Source: CAD feature listing. Evaluate the final solid. Frame: model axes, mm. Face numbers are marked on the shaded views. A direction names the side the tool comes from. Round coordinates to 2 decimals unless told otherwise and drop trailing zeros. Order: outer loops, then holes, each group sorted by start corner. A loop starts at its lowest first (then second) coordinate and runs counter-clockwise, first axis right, second up. Notation, with made-up numbers: (82, 80.25) -> (91, 80.25) arc R30 cw to (91, 108.25) -> close; hole circle Ø7 at (-28, 30). An arc over 180 degrees is marked (long way). Write item = value, one per line. Start each with the question number.
(1) Cut plane A-A on z = 22.5. Return the cut outline in (x, y) (3 decimals), then the cut area to 3 significant figures.
(2) Draft query along Y for the marked faces 4, 5 and 6. Return one class per face: released by +Y, released by -Y, zero draft, split by the parting line, or undercut.
(3) Cut plane C-C on y = 0. Return the cut outline in (x, z), then the cut area to 3 significant figures.
(4) Contact query for flat-ended pins moving along their axis: pin 1 Ø16 at (x, y) = (-2, -4.5) entering from +Z; pin 2 Ø12.5 at (x, z) = (-1, 15.5) entering from -Y; pin 3 Ø12 at (y, z) = (-6.5, 4.5) entering from +X; pin 4 Ø4 at (x, y) = (0, 16.5) entering from +Z. Output: stop coordinate, or through.
(5) Cut plane D-D on x = 0. Return the cut outline in (y, z) (3 decimals).
(6) Cut plane B-B on z = 11.75. Return the cut outline in (x, y), then the cut area to 3 significant figures.
(7) Reachability of the marked faces 1, 2 and 3 from +Z, -Z, +X, -X, +Y, -Y: full face, straight path, thin tool, end or side. Return the list, or none.
(8) Ray query, line 1 (Y direction, x = 0, z = 2.55) (3 decimals); line 2 (Z direction, x = 0, y = 23.6) (3 decimals); line 3 (Z direction, x = 0, y = -18). Return the intervals inside material, ascending.
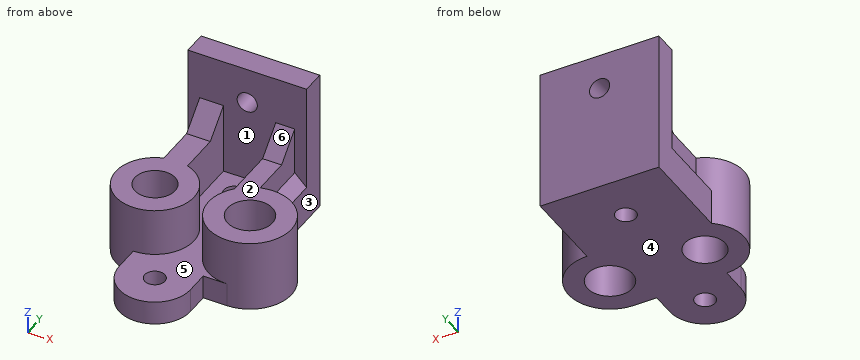
from build123d import *

# Parameters (mm, degrees)
F0_R          = 2.125
F0_R_2        = 4.25
F0_R_3        = 4.75
F1_DEPTH      = 5
F2_W          = 25
F2_H          = 5
F3_DEPTH      = 25
F4_R          = 8.25
F4_R_2        = 4.25
F4_R_3        = 8.75
F4_R_4        = 4.75
F5_DEPTH      = 10
F6_R          = 2.125
F7_DEPTH      = 5.001
F8_W          = 5
F8_H          = 13.6379074032
F8_W_2        = 4
F8_H_2        = 15.6423127431
F9_DEPTH      = 10
F10_T1_DEPTH  = 5
F10_T3_DEPTH  = 4
F10_T8_DEPTH  = 17.8584149398
F10_T13_DEPTH = 16.8584149398
F10_T18_DEPTH = 26.4963223431
F10_S19_R     = 8.25
F10_T20_DEPTH = 15
F10_T25_DEPTH = 26.4963223431
F10_S26_R     = 8.25
F10_T27_DEPTH = 15
F10_T32_DEPTH = 25.9731600242
F10_S34_R     = 8.75
F10_T35_DEPTH = 15


# Not quite as in the source:
# - a fillet or chamfer that OpenCascade refuses, or shapes differently, is made with other operations: its cross-section is extruded or revolved along the edge and cut away or added


with BuildPart() as f1:
    # F0 (on Top) → F1 (new body)
    with BuildSketch(Plane.XY):
        with BuildLine():
            Line((12.5, 26.5), (0, 26.5))
            Line((0, 26.5), (-12.5, 26.5))
            Line((-12.5, 26.5), (-12.5, 6.5622023742))
            ThreePointArc((-12.5, 6.5622023742), (-15.3166703137, -2.6385915194), (-7.5, -8.25))
            Line((-7.5, -8.25), (-7.5, -13.6))
            ThreePointArc((-7.5, -13.6), (-5.3033008589, -18.9033008589), (0, -21.1))
            ThreePointArc((0, -21.1), (5.3033008589, -18.9033008589), (7.5, -13.6))
            Line((7.5, -13.6), (7.5, -8.75))
            Line((7.5, -8.75), (12.5, -8.75))
            ThreePointArc((12.5, -8.75), (21.25, 0), (12.5, 8.75))
            Line((12.5, 8.75), (12.5, 26.5))
        make_face()
        with Locations((0, -13.6)):
            Circle(F0_R, mode=Mode.SUBTRACT)
        with Locations((-7.5, 0)):
            Circle(F0_R_2, mode=Mode.SUBTRACT)
        with Locations((12.5, 0)):
            Circle(F0_R_3, mode=Mode.SUBTRACT)
        with Locations((0, 16.5)):
            Circle(F0_R, mode=Mode.SUBTRACT)
    extrude(amount=F1_DEPTH)

    # F2 (on face) → F3 (join)
    with BuildSketch(Plane.XY.offset(5)):
        with Locations((0, 24)):
            Rectangle(F2_W, F2_H)
    extrude(amount=F3_DEPTH)

    # F4 (on face) → F5 (join)
    with BuildSketch(Plane.XY.offset(5)):
        with Locations((-7.5, 0)):
            Circle(F4_R)
        with Locations((-7.5, 0)):
            Circle(F4_R_2, mode=Mode.SUBTRACT)
        with Locations((12.5, 0)):
            Circle(F4_R_3)
        with Locations((12.5, 0)):
            Circle(F4_R_4, mode=Mode.SUBTRACT)
    extrude(amount=F5_DEPTH)

    # F6 (on face) → F7 (cut, through all)
    with BuildSketch(Plane.XZ.offset(-21.5)):
        with Locations((0, 22.5)):
            Circle(F6_R)
    extrude(amount=-F7_DEPTH, mode=Mode.SUBTRACT)

    # F8 (on face) → F9 (join)
    with BuildSketch(Plane.XY.offset(5)):
        with Locations((-7.5, 14.6810462984)):
            Rectangle(F8_W, F8_H)
        with Locations((8, 13.6788436285)):
            Rectangle(F8_W_2, F8_H_2)
    extrude(amount=F9_DEPTH)

    # F10: chamfer of 5 on 4 edges, made by hand

    # F10_s2 → F10_t1 (join)
    with BuildSketch(Plane.YZ.offset(-10)):
        Polygon((21.5, 20), (16.5, 15), (21.5, 15), align=None)
    extrude(amount=F10_T1_DEPTH)

    # F10_s4 → F10_t3 (join)
    with BuildSketch(Plane.YZ.offset(6)):
        Polygon((21.5, 20), (16.5, 15), (21.5, 15), align=None)
    extrude(amount=F10_T3_DEPTH)


with BuildPart() as f10_tool6:
    # F10_s7 → F10_t8 (new body)
    with BuildSketch(Plane.YZ.offset(7.8584149398)):
        Polygon((21.5, 20), (16.5, 15), (21.5, 15), align=None)
    extrude(amount=-F10_T8_DEPTH)

    split(bisect_by=Plane.YZ.offset(6), keep=Keep.TOP)


with BuildPart() as f1_1:
    add(f1.part)

    # F10_t5: union F10_tool6
    add(f10_tool6.part)


with BuildPart() as f10_tool11:
    # F10_s12 → F10_t13 (new body)
    with BuildSketch(Plane.YZ.offset(10)):
        Polygon((21.5, 20), (16.5, 15), (21.5, 15), align=None)
    extrude(amount=-F10_T13_DEPTH)

    split(bisect_by=Plane.YZ.offset(-5), keep=Keep.BOTTOM)


with BuildPart() as f1_2:
    add(f1_1.part)

    # F10_t10: union F10_tool11
    add(f10_tool11.part)


with BuildPart() as f10_tool16:
    # F10_s17 → F10_t18 (new body)
    with BuildSketch(Plane.XZ.offset(-21.5)):
        Polygon((-10, 10), (-15, 5), (-10, 5), align=None)
    extrude(amount=F10_T18_DEPTH)

    # F10_s19 → F10_t20 (cut, symmetric)
    with BuildSketch(Plane.XY.offset(7.5)):
        with Locations((-7.5, 0)):
            Circle(F10_S19_R)
    extrude(amount=F10_T20_DEPTH, both=True, mode=Mode.SUBTRACT)

    split(bisect_by=Plane.YZ.offset(-12.5), keep=Keep.TOP)


with BuildPart() as f1_3:
    add(f1_2.part)

    # F10_t15: union F10_tool16
    add(f10_tool16.part)


with BuildPart() as f10_tool23:
    # F10_s24 → F10_t25 (new body)
    with BuildSketch(Plane.XZ.offset(-21.5)):
        Polygon((-10, 10), (-15, 5), (-10, 5), align=None)
    extrude(amount=F10_T25_DEPTH)

    # F10_s26 → F10_t27 (intersect, symmetric)
    with BuildSketch(Plane.XY.offset(7.5)):
        with Locations((-7.5, 0)):
            Circle(F10_S26_R)
    extrude(amount=F10_T27_DEPTH, both=True, mode=Mode.INTERSECT)

    split(bisect_by=Plane.YZ.offset(-12.5), keep=Keep.BOTTOM)


with BuildPart() as f1_4:
    add(f1_3.part)

    # F10_t22: union F10_tool23
    add(f10_tool23.part)


with BuildPart() as f10_tool30:
    # F10_s31 → F10_t32 (new body)
    with BuildSketch(Plane.XZ.offset(4.4731600242)):
        Polygon((15, 5), (10, 10), (10, 5), align=None)
    extrude(amount=-F10_T32_DEPTH)

    split(bisect_by=Plane.YZ.offset(12.5), keep=Keep.BOTTOM)

    # F10_s34 → F10_t35 (cut, symmetric)
    with BuildSketch(Plane.XY.offset(7.5)):
        with Locations((12.5, 0)):
            Circle(F10_S34_R)
    extrude(amount=F10_T35_DEPTH, both=True, mode=Mode.SUBTRACT)


with BuildPart() as f1_5:
    add(f1_4.part)

    # F10_t29: union F10_tool30
    add(f10_tool30.part)


solid = f1_5.part
Evaluation:
q1.outline = (-12.5, 21.5) -> (-2.125, 21.5) -> (-2.125, 26.5) -> (-12.5, 26.5) -> close; (2.125, 21.5) -> (12.5, 21.5) -> (12.5, 26.5) -> (2.125, 26.5) -> close
q1.area = 104 mm^2
q2.face_4 = zero draft
q2.face_5 = undercut
q2.face_6 = released by -Y
q3.outline = (-15.75, 0) -> (-11.75, 0) -> (-11.75, 15) -> (-15.75, 15) -> close; (-3.25, 0) -> (7.75, 0) -> (7.75, 15) -> (3.75, 15) -> (3.75, 5) -> (0.75, 5) -> (0.75, 15) -> (-3.25, 15) -> close; (17.25, 0) -> (21.25, 0) -> (21.25, 15) -> (17.25, 15) -> close
q3.area = 255 mm^2
q4.pin_1 = 15
q4.pin_2 = -8.25
q4.pin_3 = 21.24
q4.pin_4 = through
q5.outline = (-21.1, 0) -> (-15.725, 0) -> (-15.725, 5) -> (-21.1, 5) -> close; (-11.475, 0) -> (14.375, 0) -> (14.375, 5) -> (3.437, 5) -> (3.437, 15) -> (-3.437, 15) -> (-3.437, 5) -> (-11.475, 5) -> close; (18.625, 0) -> (26.5, 0) -> (26.5, 20.375) -> (21.5, 20.375) -> (21.5, 5) -> (18.625, 5) -> close; (21.5, 24.625) -> (26.5, 24.625) -> (26.5, 30) -> (21.5, 30) -> close
q6.outline = (-12.5, 21.5) -> (-10, 21.5) -> (-10, 7.86) arc R8.25 ccw (long way) to (-5, 7.86) -> (-5, 21.5) -> (6, 21.5) -> (6, 5.86) arc R8.75 ccw (long way) to (10, 8.39) -> (10, 21.5) -> (12.5, 21.5) -> (12.5, 26.5) -> (-12.5, 26.5) -> close; hole circle Ø8.5 at (-7.5, 0); hole circle Ø9.5 at (12.5, 0)
q6.area = 575 mm^2
q7.face_1 = +Z
q7.face_2 = +Z, +X, -X, -Y
q7.face_3 = +Z, -Z, +X, +Y
q8.line_1 = -21.1 to -15.725, -11.475 to 14.375, 18.625 to 26.5
q8.line_2 = 0 to 20.375, 24.625 to 30
q8.line_3 = 0 to 5
